Here's how the part is built. I have some questions about the finished solid (model axes, mm). A direction names the side the tool comes from. Coordinates: 2 decimals unless noted, no trailing zeros. Write each loop counter-clockwise with the first axis right and the second up, starting at its lowest first coordinate (ties: lowest second). Pieces come first, ordered by that corner, then holes. Notation, with made-up numbers: (44, 42.25) -> (81, 42.25) arc R36 cw to (81, 78.25) -> close; hole circle Ø4 at (-28.75, 32.25). An arc over 180 degrees is marked (long way). Put each result on its own line as item: value. Start each with the question number.
Item 1: On a 3-axis mill with a long thin cutter (end or side, diameter ignored), from which of +Z, -Z, +X, -X, +Y, -Y can I reach the whole of each face in a straight line? I mean faces 1 (the face through (-36, 9, 66)), 2 (the face through (-44, 9, -62)), 3 (the face through (-30, 9, 67)), 4 (the face through (0, 1, 43)). Say none if no direction works.
Item 2: For pin 1 (1.5 mm diameter, centred on x = -42.5, y = 7, fed in from -Z); pin 2 (5 mm diameter, centred on x = 38.5, z = -50, fed in from -Y); pin 3 (6.5 mm diameter, centred on x = -33.5, y = 9, fed in from +Z); pin 4 (3 mm diameter, centred on x = -35, z = 73.66, fed in from +Y), each with a flat end and sliding along its axis, tell me the tip position at first contact or that it passes through.
Item 3: I need wall thicknesses on line 1 (X direction, y = 1.7, z = -65); line 2 (Z direction, x = 35, y = 1.65); line 3 (Z direction, x = 0, y = 4.15). Which ranges of each line are inside material? Lowest first, please. Write a range as [from, to].
Item 4: I want a section at D-D, the plane z = 22. List the corners of the cut face in (x, y) for me.
Item 5: If we mould it in two halves opening along X, with no side actions, what happens to faces 5 (the face through (-43, 9, 55)), 6 (the face through (44, 9, -62)), 7 (the face through (30, 9, -67))? For each: released by +X, released by -X, zero draft, split by the parting line, or undercut.
Item 6: I want a section at A-A, the plane y = 11. List the corners of the cut face in (x, z) for me.
Item 7: I want a section at B-B, the plane z = -61. List the corners of the cut face in (x, y) for me, then the cut area to 3 significant figures.
Item 8: I want a section at C-C, the plane x = -38. List the corners of the cut face in (y, z) for me, then the cut area to 3 significant figures.
from build123d import *

# Parameters (mm, degrees)
SKETCH_1_W          = 110
SKETCH_1_H          = 160
EXTRUDE_1_DEPTH     = 5
SKETCH_3_R          = 1.4
CUT_EXTRUDE_1_DEPTH = 5
EXTRUDE_2_DEPTH     = 8
SKETCH_5_R          = 3
CUT_EXTRUDE_2_DEPTH = 2.5


with BuildPart() as part:
    # 스케치1 → 보스-돌출1 (new body)
    with BuildSketch(Plane(origin=(0, 0, 0), x_dir=(1, 0, 0), z_dir=(0, 1, 0))):
        Rectangle(SKETCH_1_W, SKETCH_1_H)
    extrude(amount=EXTRUDE_1_DEPTH)

    # 스케치3 → 컷-돌출1 (cut)
    with BuildSketch(Plane(origin=(0, 5, 0), x_dir=(1, 0, 0), z_dir=(0, 1, 0))):
        with Locations((-50, 65)):
            Circle(SKETCH_3_R)
        with Locations((-45, 73.660254038)):
            Circle(SKETCH_3_R)
        with Locations((-35, 73.660254038)):
            Circle(SKETCH_3_R)
        with Locations((-50, -65)):
            Circle(SKETCH_3_R)
        with Locations((-45, -73.660254038)):
            Circle(SKETCH_3_R)
        with Locations((-35, -73.660254038)):
            Circle(SKETCH_3_R)
        with Locations((35, 73.660254038)):
            Circle(SKETCH_3_R)
        with Locations((45, 73.660254038)):
            Circle(SKETCH_3_R)
        with Locations((50, 65)):
            Circle(SKETCH_3_R)
        with Locations((35, -73.660254038)):
            Circle(SKETCH_3_R)
        with Locations((45, -73.660254038)):
            Circle(SKETCH_3_R)
        with Locations((50, -65)):
            Circle(SKETCH_3_R)
        with Locations((0, 40)):
            Circle(SKETCH_3_R)
        with Locations((0, -40)):
            Circle(SKETCH_3_R)
    extrude(amount=-CUT_EXTRUDE_1_DEPTH, mode=Mode.SUBTRACT)

    # 스케치4 → 보스-돌출2 (add)
    with BuildSketch(Plane(origin=(0, 5, 0), x_dir=(1, 0, 0), z_dir=(0, 1, 0))):
        Polygon((41, 66), (30, 66), (30, 69), (44, 69), (44, 55), (41, 55), align=None)
        Polygon((44, -55), (41, -55), (41, -66), (30, -66), (30, -69), (44, -69), align=None)
        Polygon((-44, 55), (-41, 55), (-41, 66), (-30, 66), (-30, 69), (-44, 69), align=None)
        Polygon((-44, -55), (-41, -55), (-41, -66), (-30, -66), (-30, -69), (-44, -69), align=None)
    extrude(amount=EXTRUDE_2_DEPTH)

    # 스케치5 → 컷-돌출2 (cut)
    with BuildSketch(Plane.XZ):
        with Locations((0, 40)):
            Circle(SKETCH_5_R)
        with Locations((0, -40)):
            Circle(SKETCH_5_R)
    extrude(amount=-CUT_EXTRUDE_2_DEPTH, mode=Mode.SUBTRACT)


solid = part.part
Calculated:
1. face 1: +Y
1. face 2: +Z, -Z, -X, +Y
1. face 3: +Z, -Z, +Y
1. face 4: -Y
2. pin 1: stops at z = -69
2. pin 2: stops at y = 0
2. pin 3: stops at z = 69
2. pin 4: stops at y = 5
3. line 1: x = [-55, -51.4], [-48.6, 48.6], [51.4, 55]
3. line 2: z = [-80, -75.06], [-72.26, 72.26], [75.06, 80]
3. line 3: z = [-80, -41.4], [-38.6, 38.6], [41.4, 80]
4. outline: (-55, 0) -> (55, 0) -> (55, 5) -> (-55, 5) -> close
5. face 5: zero draft
5. face 6: released by +X
5. face 7: undercut
6. outline: (-44, -69) -> (-30, -69) -> (-30, -66) -> (-41, -66) -> (-41, -55) -> (-44, -55) -> close; (-44, 55) -> (-41, 55) -> (-41, 66) -> (-30, 66) -> (-30, 69) -> (-44, 69) -> close; (30, -69) -> (44, -69) -> (44, -55) -> (41, -55) -> (41, -66) -> (30, -66) -> close; (30, 66) -> (41, 66) -> (41, 55) -> (44, 55) -> (44, 69) -> (30, 69) -> close
7. outline: (-55, 0) -> (55, 0) -> (55, 5) -> (44, 5) -> (44, 13) -> (41, 13) -> (41, 5) -> (-41, 5) -> (-41, 13) -> (-44, 13) -> (-44, 5) -> (-55, 5) -> close
7. area: 598 mm2
8. outline: (0, -80) -> (5, -80) -> (5, -69) -> (13, -69) -> (13, -66) -> (5, -66) -> (5, 66) -> (13, 66) -> (13, 69) -> (5, 69) -> (5, 80) -> (0, 80) -> close
8. area: 848 mm2
